Autodesk Inventor part; units mm, degrees
ref_plane "YZ Plane" through (0, 0, 0) normal (1, 0, 0) x (0, 1, 0)
ref_plane "XZ Plane" through (0, 0, 0) normal (0, 1, 0) x (-1, 0, 0)
ref_plane "XY Plane" through (0, 0, 0) normal (0, 0, 1) x (1, 0, 0)
sketch "Sketch1" plane through (0, 0, 0) normal (0, 0, 1) x (1, 0, 0)
  line L0 (5.5, -5) -> (-5.5, -5) construction
  line L1 (-5.5, -5) -> (-5.5, 5)
  line L2 (-5.5, 5) -> (5.5, 5)
  line L3 (5.5, 5) -> (5.5, -5)
  line L4 (5.5, -5) -> (-5.5, 5) construction
  line L5 (-5.5, -5) -> (5.5, 5) construction
  line L6 (-7.5, 7) -> (7.5, 7)
  line L7 (7.5, 7) -> (7.5, -5)
  line L8 (7.5, -5) -> (-7.5, -5)
  line L9 (-7.5, -5) -> (-7.5, 7)
  line L10 (0, 0) -> (0, 7) construction
  point P0 (0, 0)
  dimension "d6" = 11
  dimension "d7" = 10
  dimension "d8" = 2
  dimension "d9" = 10
  dimension "d10" = 2
extrude "Extrusion1" add sketch "Sketch1" along normal blind 30 contours L8 L9 L6 L7 L3 L2 L1
sketch "Sketch2" plane through (-7.5, 7, 0) normal (0, 1, 0) x (1, 0, 0)
  line L0 (7.5, 0) -> (7.5, -30) construction
  line L1 (15, -30) -> (0, -30) construction
  circle A0 centre (7.5, -22.1) radius 4.15
  dimension "d14" = 7.9
  dimension "d15" = 8.3
extrude "Extrusion2" cut sketch "Sketch2" against normal up to next
sketch "Sketch3" plane through (0, 0, 0) normal (0, 0, 1) x (1, 0, 0)
  line L0 (-7.5, 7) -> (-7.5, -5) construction
  line L1 (7.5, -5) -> (7.5, 7) construction
  line L2 (5.5, -5) -> (7.5, -5) construction
  line L3 (7.5, 7) -> (-7.5, 7) construction
  line L4 (-7.5, -5) -> (-5.5, -5) construction
  line L5 (5.5, 5) -> (5.5, -5) construction
  line L6 (-5.5, -5) -> (5.5, -5) construction
  line L7 (0, -5) -> (0, 7)
  line L8 (-4.15, 7) -> (4.15, 7) construction
  line L9 (-7.5, 7) -> (-7.5, -5) construction
  line L10 (-7.5, 0) -> (7.5, 0)
  point P0 (0, 0)
fillet "Fillet1" radius 1 6 edges at (-5.5, -5, 15) (-7.5, -5, 15) (5.5, -5, 15) (7.5, -5, 15) (-5.5, 5, 15) (5.5, 5, 15)
fillet "Fillet4" radius 3 2 edges at (-7.5, 7, 15) (7.5, 7, 15)
properties part number "base_fotodiode"
Source: CAD feature listing. Evaluate the final solid. Frame: model axes, mm. A direction names the side the tool comes from. Round coordinates to 2 decimals unless told otherwise and drop trailing zeros. Loops run counter-clockwise (first coordinate to the right, second up) from the corner with the lowest first, then second, coordinate; pieces in that order, holes last. Notation, with made-up numbers: M 87,84.25 L 97,84.25 A23 cw 97,95.25 Z; hole C 18,2.25 d8. An arc over 180 degrees is marked long. Return JSON: item names as keys, results as strings. Group by question number.
1. Mould query, pull axis X, two halves, no side actions, for faces 1 (the face through (5.785, -4.699, 15.21)), 2 (the face through (7.199, -4.715, 15.21)), 3 (the face through (0, 7, 11)), 4 (the face through (-7.5, 0, 15)). Classes: released by +X, released by -X, zero draft, split by the parting line, or undercut.
2. Reachability of faces 5 (the face through (0, 6, 0)), 6 (the face through (5.5, 0, 15)) from +Z, -Z, +X, -X, +Y, -Y: full face, straight path, thin tool, end or side. Return the list, or none.
3. Section query B-B on x = 0. Output: boundary loops of the cut face in (y, z), and give its area (3 significant figures).
4. Pin query (flat end, axial travel): pin 1 (3 mm diameter, centred on x = 2.5, y = 1.5, fed in from -Z); pin 2 (6 mm diameter, centred on x = -3, z = 13, fed in from -Y); pin 3 (8 mm diameter, centred on x = 0, z = 12.5, fed in from -Y). Return the tip coordinate at first contact, or that it passes through.
5. Section query C-C on y = -0.75. Output: boundary loops of the cut face in (x, z).
6. Material intervals for line 1 along X through (y, z) = (0, 19.25); line 2 along Z through (x, y) = (0, 6); line 3 along Z through (x, y) = (1.25, 5.5), sorted ascending. Write a range as from..to.
Checks:
{
 "1": {"face 1": "undercut", "face 2": "released by +X", "face 3": "zero draft", "face 4": "released by -X"},
 "2": {"face 5": "-Z, +X, -X, +Y, -Y", "face 6": "+Z, -Z, -Y"},
 "3": {"outline": "M 5,0 L 7,0 L 7,17.95 L 5,17.95 Z; M 5,26.25 L 7,26.25 L 7,30 L 5,30 Z", "area": "43.4 mm²"},
 "4": {"pin 1": "passes through", "pin 2": "stops at y = -4.87", "pin 3": "stops at y = 5"},
 "5": {"outline": "M -7.5,0 L -5.5,0 L -5.5,30 L -7.5,30 Z; M 5.5,0 L 7.5,0 L 7.5,30 L 5.5,30 Z"},
 "6": {"line 1": "x = -7.5..-5.5, 5.5..7.5", "line 2": "z = 0..17.95, 26.25..30", "line 3": "z = 0..18.14, 26.06..30"}
}
